```python
from build123d import *

# Parameters (mm, degrees)
F1_DEPTH = 50
F2_R     = 20
F3_DEPTH = 40
F5_D     = 20
F6_R     = 24.99999
F8_D     = 20
F8_DEPTH = 40.001
F10_D    = 20


# Not quite as in the source:
# - a fillet or chamfer is up to 0.001 mm smaller than in the source, because OpenCascade refuses the exact size


with BuildPart() as f1:
    # F0 (on Front) → F1 (new body)
    with BuildSketch(Plane.XZ):
        Polygon((-25, 80), (-25, 0), (25, 0), (25, 80), (12.5, 80), (12.5, 15), (0, 15), (-12.5, 15), (-12.5, 80), align=None)
    extrude(amount=F1_DEPTH)

    # F2 (on face) → F3 (join)
    with BuildSketch(Plane(origin=(0, 0, 0), x_dir=(1, 0, 0), z_dir=(0, 0, -1))):
        with Locations((0, 25)):
            Circle(F2_R)
    extrude(amount=F3_DEPTH)

    # F5 (through all)
    with Locations(Plane.YZ.offset(25)):
        with Locations((-25, 55)):
            Hole(F5_D / 2)

    # F6 (radius 25 in the source; OpenCascade refuses exactly that, so slightly less here)
    f6_edges = [f1.edges().sort_by_distance(p)[0] for p in [
        (18.75, -50, 80),
        (18.75, 0, 80),
        (-18.75, -50, 80),
        (-18.75, 0, 80),
    ]]
    fillet(f6_edges, radius=F6_R)

    # F8 (through all, one way)
    with BuildSketch(Plane.XY):
        with Locations((0, -25)):
            Circle(F8_D / 2)
    extrude(amount=-F8_DEPTH, mode=Mode.SUBTRACT)

    # F10 (through all)
    with Locations(Plane.XY.offset(15)):
        with Locations((0, -25)):
            Hole(F10_D / 2)


solid = f1.part
```
Source: CAD feature listing. Evaluate the final solid. Frame: model axes, mm. A direction names the side the tool comes from. Round coordinates to 2 decimals unless told otherwise and drop trailing zeros. Order: outer loops, then holes, each group sorted by start corner. A loop starts at its lowest first (then second) coordinate and runs counter-clockwise, first axis right, second up. Notation, with made-up numbers: (-20.75, 29) -> (-4.75, 29) arc R24 ccw to (-4.75, 40) -> close; hole circle Ø10 at (13.25, -38). An arc over 180 degrees is marked (long way). One line per item, written item: value. Start each with the question number.
Q1. Section query C-C (y = -23.5). Return the cut outline in (x, z), plus the area to 3 significant figures.
Q2. Section query B-B (x = 0). Return the cut outline in (y, z), plus the area to 3 significant figures.
Q3. Material intervals for probe 1 along Z at (x, y) = (21.75, -25); probe 2 along X at (y, z) = (-39, 30.5); probe 3 along Y at (x, z) = (0, 11.75), sorted ascending.
Q4. Draft query along X for faces 4 (the flat face through (-12.5, -25, 40)), 5 (the cylindrical face through (-4.336, -5.476, -19.72)), 6 (the flat face through (-25, -25, 41)), 7 (the cylindrical face through (-18.838, -29.614, 46.128)). Return one class per face: pulls with the +X half, pulls with the -X half, needs draft (parallel to the pull), parting line crosses it, or undercut.
Q5. Access query for faces 1 (the flat face through (0, -50, 10)), 2 (the flat face through (9, -19, 15)), 3 (the flat face through (-17, -14, 0)). Directions: +Z, -Z, +X, -X, +Y, -Y. A direction counts if a zero-diameter tool reaches every point of the face in a straight line with its end or side. Return the directions, or none.
Q6. Section query D-D (z = 56.5). Return the cut outline in (x, y).
Q7. Pin query (flat end, axial travel): pin 1 (12 mm diameter, centred on x = 5, y = -15, fed in from +Z); pin 2 (8 mm diameter, centred on x = -10.5, y = -15, fed in from +Z); pin 3 (18 mm diameter, centred on x = 0, y = -25, fed in from -Z); pin 4 (1.5 mm diameter, centred on x = -17.5, y = -16.5, fed in from +Z). Return the tip coordinate at first contact, or that it passes through.
Q8. Section query A-A (z = 40.5). Return the cut outline in (x, y), plus the area to 3 significant figures.
Findings below:
1. outline: (-25, 0) -> (-19.94, 0) -> (-19.94, -40) -> (-9.89, -40) -> (-9.89, 15) -> (-12.5, 15) -> (-12.5, 45.11) -> (-25, 45.11) -> close; (-25, 64.89) -> (-12.5, 64.89) -> (-12.5, 79.95) -> (-25, 79.95) -> close; (9.89, -40) -> (19.94, -40) -> (19.94, 0) -> (25, 0) -> (25, 45.11) -> (12.5, 45.11) -> (12.5, 15) -> (9.89, 15) -> close; (12.5, 64.89) -> (25, 64.89) -> (25, 79.95) -> (12.5, 79.95) -> close
1. area: 2,390 mm²
2. outline: (-50, 0) -> (-45, 0) -> (-45, -40) -> (-35, -40) -> (-35, 15) -> (-50, 15) -> close; (-15, -40) -> (-5, -40) -> (-5, 0) -> (0, 0) -> (0, 15) -> (-15, 15) -> close
2. area: 1,250 mm²
3. probe 1: 0 to 45, 65 to 80
3. probe 2: -25 to -12.5, 12.5 to 25
3. probe 3: -50 to -35, -15 to 0
4. face 4: undercut
4. face 5: parting line crosses it
4. face 6: pulls with the -X half
4. face 7: needs draft
5. face 1: +Z, -Z, +X, -X, -Y
5. face 2: +Z, +Y, -Y
5. face 3: -Z
6. outline: (-25, -49.95) -> (-12.5, -49.95) -> (-12.5, -34.89) -> (-25, -34.89) -> close; (-25, -15.11) -> (-12.5, -15.11) -> (-12.5, -0.05) -> (-25, -0.05) -> close; (12.5, -49.95) -> (25, -49.95) -> (25, -34.89) -> (12.5, -34.89) -> close; (12.5, -15.11) -> (25, -15.11) -> (25, -0.05) -> (12.5, -0.05) -> close
7. pin 1: z = 15
7. pin 2: z = 79.13
7. pin 3: through
7. pin 4: z = 78.77
8. outline: (-25, -50) -> (-12.5, -50) -> (-12.5, 0) -> (-25, 0) -> close; (12.5, -50) -> (25, -50) -> (25, 0) -> (12.5, 0) -> close
8. area: 1,250 mm²
